Design review of the part built by this model. Coordinates are the model's own, in mm. Face numbers are marked on the shaded views. A direction names the side the tool comes from. Coordinates: 2 decimals unless noted, no trailing zeros. Order: outer loops, then holes, each group sorted by start corner. A loop starts at its lowest first (then second) coordinate and runs counter-clockwise, first axis right, second up.
from build123d import *

# Parameters (mm, degrees)
F1_DEPTH = 28.575
F2_W     = 73.406
F2_H     = 28.448
F3_DEPTH = 14.2875
F5_DEPTH = 26.741029


with BuildPart() as f1:
    # F0 (on Top) → F1 (new body)
    with BuildSketch(Plane.XY):
        Polygon((0, -14.389101), (28.583242, -14.389101), (28.583242, 11.010899), (0, 11.010899), (0, 5.581491), (-69.596, 5.581491), (-69.596, -4.133693), (-63.246, -4.133693), (-63.246, -8.959693), (0, -8.959693), align=None)
    extrude(amount=F1_DEPTH)

    # F2 (on Top) → F3 (join)
    with BuildSketch(Plane.XY):
        with Locations((-32.863217, -1.873072)):
            Rectangle(F2_W, F2_H)
    extrude(amount=-F3_DEPTH)

    # F4 (on face) → F5 (cut, through all)
    with BuildSketch(Plane.XZ.offset(14.389101)):
        Polygon((28.583242, 0), (28.583242, 28.575), (0.008242, 0), (3.839783, 0), align=None)
    extrude(amount=-F5_DEPTH, mode=Mode.SUBTRACT)


solid = f1.part
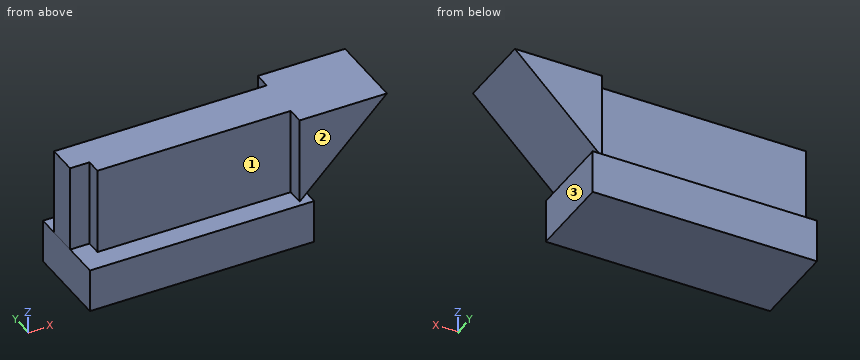
1. Insertion check: pin 1 (14.5 mm diameter, centred on x = -23, z = 11, fed in from +Y); pin 2 (1 mm diameter, centred on y = -9.5, z = 22, fed in from -X); pin 3 (23 mm diameter, centred on x = 12.5, z = 12, fed in from -Y). Each pin has a flat end and moves straight along its axis. Give the tip position at first contact, or say it passes through.
2. Add section B-B (x = -27). Give the boundary of the cut face in (y, z) (1 decimal).
3. Add section C-C (z = 26). Give the boundary of the cut face in (x, y).
4. Add section A-A (y = 10). Give the boundary of the cut face in (x, z) (1 decimal).
5. To check wall thickness, follow line 1 (Z direction, x = -45, y = -10); line 2 (Y direction, x = 3, z = 4); line 3 (X direction, y = 3.5, z = -6.5). State the ranges of each line that lie inside material, in increasing order.
6. Add section D-D (z = 18.5). Give the boundary of the cut face in (x, y), and give its area (3 significant figures).
7. For the marked faces 1, 2 and 3, list the 3-axis set-ups (+Z, -Z, +X, -X, +Y, -Y) from which the entire face can be reached by the end or side of a thin tool; tool diameter is ignored.
Solution:
1. pin 1: stops at y = 5.58
1. pin 2: stops at x = 0
1. pin 3: stops at y = -14.39
2. outline: (-16.1, -14.3) - (12.4, -14.3) - (12.4, 0) - (5.6, 0) - (5.6, 28.6) - (-9, 28.6) - (-9, 0) - (-16.1, 0) - close
3. outline: (-69.6, -4.13) - (-63.25, -4.13) - (-63.25, -8.96) - (0, -8.96) - (0, -14.39) - (26.01, -14.39) - (26.01, 11.01) - (0, 11.01) - (0, 5.58) - (-69.6, 5.58) - close
4. outline: (-69.6, -14.3) - (3.8, -14.3) - (3.8, 0) - (0, 0) - (28.6, 28.6) - (0, 28.6) - (0, 0) - (-69.6, 0) - close
5. line 1: z = -14.29 to 0
5. line 2: y = -14.39 to 11.01
5. line 3: x = -69.57 to 3.84
6. outline: (-69.6, -4.13) - (-63.25, -4.13) - (-63.25, -8.96) - (0, -8.96) - (0, -14.39) - (18.51, -14.39) - (18.51, 11.01) - (0, 11.01) - (0, 5.58) - (-69.6, 5.58) - close
6. area: 1,450 mm2
7. face 1: +Z, -X, -Y
7. face 2: +Z, +X, -X, -Y
7. face 3: -Z, +X, +Y, -Y
